from build123d import *

# Parameters (mm, degrees)
CROQUIS1_W              = 10
CROQUIS1_H              = 10
SALIENTE_EXTRUIR1_DEPTH = 15
REDONDEO1_R             = 1
CROQUIS4_R              = 1.5
SALIENTE_EXTRUIR2_DEPTH = 7.5
CROQUIS5_R              = 1.5
SALIENTE_EXTRUIR3_DEPTH = 7.5


with BuildPart() as part:
    # Croquis1 → Saliente-Extruir1 (new body)
    with BuildSketch(Plane.XY):
        Rectangle(CROQUIS1_W, CROQUIS1_H)
    extrude(amount=SALIENTE_EXTRUIR1_DEPTH)

    # Croquis3 → Cortar-Revoluci_n1 (revolve, cut)
    with BuildSketch(Plane(origin=(0, 0, 0), x_dir=(0, 0, -1), z_dir=(1, 0, 0)), mode=Mode.PRIVATE) as cortar_revoluci_n1_sk:
        Polygon((-15, 4.75), (-15, 15.04), (0, 15.04), (0, 4.75), (-4.474464586, 12.5), (-10.525535414, 12.5), align=None)
    revolve(cortar_revoluci_n1_sk.sketch.rotate(Axis((0, 0, -0.75), (0, 0, 1)), 314.999999855), axis=Axis((0, 0, -0.75), (0, 0, 1)), mode=Mode.SUBTRACT)

    # Redondeo1
    # the kernel refuses this fillet: 1 mm, written as the material it takes off along each edge
    with BuildSketch(Plane(origin=(-5, 5, -1.159930874), x_dir=(1, 0, 0), z_dir=(0, 0, 1)), Plane(origin=(-5, -5, -1.159930874), x_dir=(0, 1, 0), z_dir=(0, 0, 1))) as redondeo1_piece_1:
        with BuildLine():
            CenterArc((REDONDEO1_R, -REDONDEO1_R), REDONDEO1_R, 90, 90)
            Line((0, -REDONDEO1_R), (0, 0))
            Line((0, 0), (REDONDEO1_R, 0))
        make_face()
    extrude(amount=17.319861748, mode=Mode.SUBTRACT)
    with BuildSketch(Plane(origin=(5, -5, -1.159930874), x_dir=(0, 1, 0), z_dir=(0, 0, 1)), Plane(origin=(5, 5, -1.159930874), x_dir=(-1, 0, 0), z_dir=(0, 0, 1))) as redondeo1_piece_2:
        with BuildLine():
            CenterArc((REDONDEO1_R, REDONDEO1_R), REDONDEO1_R, 180, 90)
            Line((0, REDONDEO1_R), (0, 0))
            Line((0, 0), (REDONDEO1_R, 0))
        make_face()
    extrude(amount=17.319861748, mode=Mode.SUBTRACT)

    # Croquis4 → Saliente-Extruir2 (add, symmetric)
    with BuildSketch(Plane(origin=(0, 0, 0), x_dir=(0, 0, -1), z_dir=(1, 0, 0))):
        with Locations(Location((-3, 0, 0), (0, 0, 90))):
            Circle(CROQUIS4_R)
    extrude(amount=SALIENTE_EXTRUIR2_DEPTH, both=True)

    # Croquis5 → Saliente-Extruir3 (add, symmetric)
    with BuildSketch(Plane(origin=(0, 0, 0), x_dir=(1, 0, 0), z_dir=(0, 1, 0))):
        with Locations(Location((0, -12, 0), (0, 0, 270))):
            Circle(CROQUIS5_R)
    extrude(amount=SALIENTE_EXTRUIR3_DEPTH, both=True)


solid = part.part
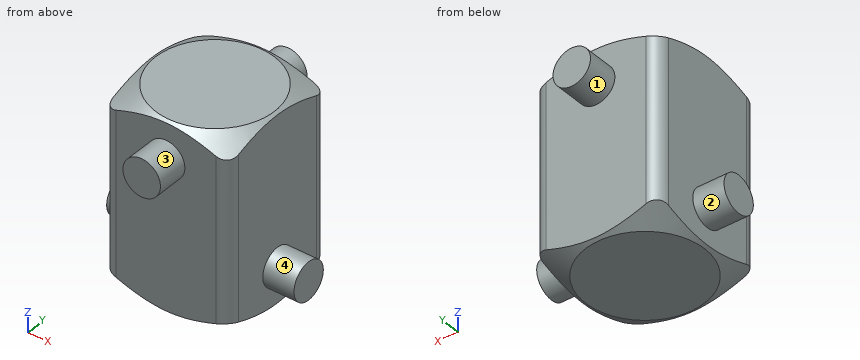
Could you check a few things on this model? Use its own coordinates, in mm. Face numbers are marked on the shaded views. A direction names the side the tool comes from. Give positions to 0.01 mm unless a question says otherwise; leave off trailing zeros. Order: outer loops, then holes, each group sorted by start corner. A loop starts at its lowest first (then second) coordinate and runs counter-clockwise, first axis right, second up. Notation, with made-up numbers: (-19.5, 34.25) - (22.5, 34.25) arc R23 ccw to (22.5, 55.25) - close; hole circle Ø4 at (76, 57.25). An arc over 180 degrees is marked (long way). Return JSON: item names as keys, results as strings. Group by question number.
Q1. Suppose I cut it at B-B, the plane x = 0. Please give me the cut outline in (y, z).
Q2. Suppose I cut it at C-C, the plane y = -5.5. Please give me the cut outline in (x, z).
Q3. Suppose I cut it at D-D, the plane z = 5.25. Please give me the cut outline in (x, y), and give its area (3 significant figures).
Q4. Which directions (+Z, -Z, +X, -X, +Y, -Y) give clear straight access to the entire face, cutting with the end or side of a thin tool? Please do the marked faces 1, 2, 3 and 4.
Q5. Will these pins go through, and if not, where does the flat tip stop? pin 1 Ø5 at (x, z) = (5, 11) entering from -Y; pin 2 Ø2.5 at (y, z) = (-0.5, 9.5) entering from -X; pin 3 Ø4 at (y, z) = (-1.5, 9.5) entering from +X.
Q6. Suppose I cut it at A-A, the plane z = 3. Please give me the cut outline in (x, y).
Q7. Please list where these lines run through material, in increasing order: line 1 along Y through (x, z) = (-3, 13.75); line 2 along Z through (x, y) = (-5.5, 0). Write a range as [from, to].
Resolved:
{
 "1": {"outline": "(-7.5, 10.5) - (-5, 10.5) - (-5, 0.14) - (-4.75, 0) - (4.75, 0) - (5, 0.14) - (5, 10.5) - (7.5, 10.5) - (7.5, 13.5) - (5, 13.5) - (5, 14.86) - (4.75, 15) - (-4.75, 15) - (-5, 14.86) - (-5, 13.5) - (-7.5, 13.5) - close"},
 "2": {"outline": "circle Ø3 at (0, 12)"},
 "3": {"outline": "(-5, -4) arc R1 ccw to (-4, -5) - (4, -5) arc R1 ccw to (5, -4) - (5, 4) arc R1 ccw to (4, 5) - (-4, 5) arc R1 ccw to (-5, 4) - close", "area": "99.1 mm2"},
 "4": {"face 1": "+Y", "face 2": "-X", "face 3": "-Y", "face 4": "+X"},
 "5": {"pin 1": "stops at y = -5", "pin 2": "stops at x = -5", "pin 3": "stops at x = 5"},
 "6": {"outline": "(-7.5, -1.5) - (-5, -1.5) - (-5, -4) arc R1 ccw to (-4, -5) - (4, -5) arc R1 ccw to (5, -4) - (5, -1.5) - (7.5, -1.5) - (7.5, 1.5) - (5, 1.5) - (5, 4) arc R1 ccw to (4, 5) - (-4, 5) arc R1 ccw to (-5, 4) - (-5, 1.5) - (-7.5, 1.5) - close"},
 "7": {"line 1": "y = [-5, 5]", "line 2": "z = [1.5, 4.5]"}
}
